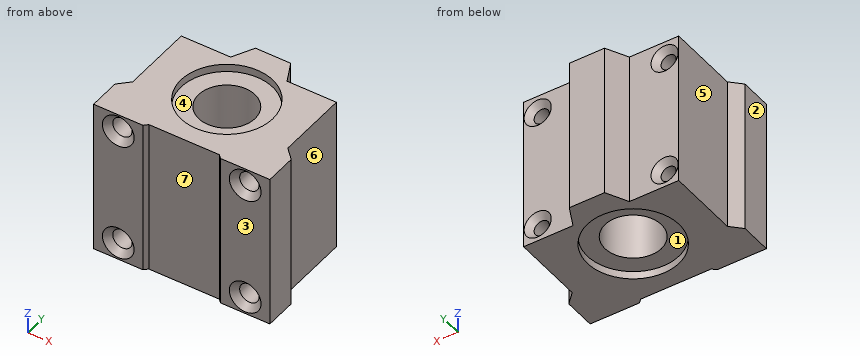
from build123d import *

# Parameters (mm, degrees)
ESBO_O1_R                                            = 8
EXTRUS_O1_DEPTH                                      = 44
ESBO_O2_R                                            = 13
EXTRUS_O2_DEPTH                                      = 2.2
ESBO_O3_R                                            = 13
EXTRUS_O3_DEPTH                                      = 2.2
ESBO_O4_R                                            = 2.15
EXTRUS_O4_DEPTH                                      = 33.5
ESCAREADO_PARA_PARAFUSO_DE_M_QUINA_COM_C_D           = 5.5
ESCAREADO_PARA_PARAFUSO_DE_M_QUINA_COM_C_DEPTH       = 12
ESCAREADO_PARA_PARAFUSO_DE_M_QUINA_COM_C_CSINK_D     = 9
ESCAREADO_PARA_PARAFUSO_DE_M_QUINA_COM_C_CSINK_ANGLE = 90
ESCAREADO_PARA_PARAFUSO_DE_M_QUINA_COM_C_TIP         = 1.652366702
CHANFRO1_SIZE                                        = 1.7


with BuildPart() as part:
    # Esboço1 → Extrusão1 (new body)
    with BuildSketch(Plane.XY):
        Polygon((-22, 13.5), (-22, -7), (-25, -10), (-25, -19), (-11, -19), (-10, -18), (10, -18), (11, -19), (25, -19), (25, -10), (22, -7), (22, 13.5), (8, 13.5), (5, 19.5), (-5, 19.5), (-8, 13.5), align=None)
        Circle(ESBO_O1_R, mode=Mode.SUBTRACT)
    extrude(amount=EXTRUS_O1_DEPTH)

    # Esboço2 → Extrusão2 (cut)
    with BuildSketch(Plane.XY.offset(44)):
        Circle(ESBO_O2_R)
    extrude(amount=-EXTRUS_O2_DEPTH, mode=Mode.SUBTRACT)

    # Esboço3 → Extrusão3 (cut)
    with BuildSketch(Plane(origin=(0, 0, 0), x_dir=(-1, 0, 0), z_dir=(0, 0, -1))):
        Circle(ESBO_O3_R)
    extrude(amount=-EXTRUS_O3_DEPTH, mode=Mode.SUBTRACT)

    # Esboço4 → Extrusão4 (cut, through all)
    with BuildSketch(Plane(origin=(0, 13.5, 0), x_dir=(1, 0, 0), z_dir=(0, 1, 0))):
        with Locations((18, -5)):
            Circle(ESBO_O4_R)
        with Locations((18, -39)):
            Circle(ESBO_O4_R)
        with Locations((-18, -5)):
            Circle(ESBO_O4_R)
        with Locations((-18, -39)):
            Circle(ESBO_O4_R)
    extrude(amount=-EXTRUS_O4_DEPTH, mode=Mode.SUBTRACT)

    # Escareado para parafuso de máquina com cabeça chata de M52
    with Locations(Plane(origin=(-18, -19, 39), x_dir=(-1, 0, 0), z_dir=(0, -1, 0))):
        with Locations((0, 0), (0, 34), (-36, 34), (-36, 0)):
            CounterSinkHole(ESCAREADO_PARA_PARAFUSO_DE_M_QUINA_COM_C_D / 2, ESCAREADO_PARA_PARAFUSO_DE_M_QUINA_COM_C_CSINK_D / 2, depth=ESCAREADO_PARA_PARAFUSO_DE_M_QUINA_COM_C_DEPTH, counter_sink_angle=ESCAREADO_PARA_PARAFUSO_DE_M_QUINA_COM_C_CSINK_ANGLE)
            with Locations((0, 0, -(ESCAREADO_PARA_PARAFUSO_DE_M_QUINA_COM_C_DEPTH + ESCAREADO_PARA_PARAFUSO_DE_M_QUINA_COM_C_TIP / 2))):  # 118° drill point
                Cone(0, ESCAREADO_PARA_PARAFUSO_DE_M_QUINA_COM_C_D / 2, ESCAREADO_PARA_PARAFUSO_DE_M_QUINA_COM_C_TIP, mode=Mode.SUBTRACT)

    # Chanfro1
    chanfro1_edges = [part.edges().sort_by_distance(p)[0] for p in [
        (15.85, 13.5, 5),
        (15.85, 13.5, 39),
        (-20.15, 13.5, 5),
        (-20.15, 13.5, 39),
    ]]
    chamfer(chanfro1_edges, length=CHANFRO1_SIZE)


solid = part.part
Part model, mm, in its own coordinate system. Face numbers are marked on the shaded views. A direction names the side the tool comes from. Round coordinates to 2 decimals unless told otherwise and drop trailing zeros. Write each loop counter-clockwise with the first axis right and the second up, starting at its lowest first coordinate (ties: lowest second). Pieces come first, ordered by that corner, then holes. Notation, with made-up numbers: M -3.75,-33 L 47.25,-33 A11 cw 47.25,-25 Z; hole C -23.75,49.5 d5. An arc over 180 degrees is marked long. Return JSON: item names as keys, results as strings. Group by question number.
(1) Saw through at C-C on z = 31. Write the cut outline in (x, y), then the cut area to 3 significant figures.
(2) Drill centre lines: probe 1 along Z at (x, y) = (18, 3); probe 2 along X at (y, z) = (-11, 39); probe 3 along X at (y, z) = (6, 5). Where is each one in solid material? Low to high.
(3) Pin check, flat tips, straight feed: pin 1 Ø1 at (x, z) = (17.5, 24.5) entering from +Y; pin 2 Ø8 at (x, y) = (18, 3.5) entering from -Z; pin 3 Ø1 at (x, y) = (11.5, -1) entering from -Z; pin 4 Ø5 at (x, z) = (-18, 39) entering from -Y. Stop position of each tip, or through.
(4) Two-plate mould, pull along Y, no slides. Class the marked faces 1, 2, 3 and 4: +Y half, -Y half, draft (parallel to the pull), parting line (faces both ways), or undercut.
(5) Saw through at A-A on y = 0. Write the cut outline in (x, z), then the cut area to 3 significant figures.
(6) Saw through at D-D on x = 0. Write the cut outline in (y, z), then the cut area to 3 significant figures.
(7) Saw through at B-B on x = 18. Write the cut outline in (y, z).
(8) Which spindle directions (+Z, -Z, +X, -X, +Y, -Y) get a long thin tool onto all of the face, cutting with end or side? Do the marked faces 5, 6 and 7. Say none if no direction does.
Returned:
{
 "1": {"outline": "M -25,-19 L -11,-19 L -10,-18 L 10,-18 L 11,-19 L 25,-19 L 25,-10 L 22,-7 L 22,13.5 L 8,13.5 L 5,19.5 L -5,19.5 L -8,13.5 L -22,13.5 L -22,-7 L -25,-10 Z; hole C 0,0 d16", "area": "1,350 mm²"},
 "2": {"probe 1": "0 to 2.85, 7.15 to 36.85, 41.15 to 44", "probe 2": "-25 to -20.75, -15.25 to 15.25, 20.75 to 25", "probe 3": "-22 to -20.15, -15.85 to -5.29, 5.29 to 15.85, 20.15 to 22"},
 "3": {"pin 1": "y = 13.5", "pin 2": "z = 0", "pin 3": "z = 2.2", "pin 4": "y = -6.85"},
 "4": {"face 1": "undercut", "face 2": "draft", "face 3": "-Y half", "face 4": "undercut"},
 "5": {"outline": "M -22,0 L -13,0 L -13,2.2 L -8,2.2 L -8,41.8 L -13,41.8 L -13,44 L -22,44 Z; M 8,2.2 L 13,2.2 L 13,0 L 22,0 L 22,44 L 13,44 L 13,41.8 L 8,41.8 Z; hole C -18,5 d4.3; hole C -18,39 d4.3; hole C 18,5 d4.3; hole C 18,39 d4.3", "area": "1,130 mm²"},
 "6": {"outline": "M -18,0 L -13,0 L -13,2.2 L -8,2.2 L -8,41.8 L -13,41.8 L -13,44 L -18,44 Z; M 8,2.2 L 13,2.2 L 13,0 L 19.5,0 L 19.5,44 L 13,44 L 13,41.8 L 8,41.8 Z", "area": "902 mm²"},
 "7": {"outline": "M -19,0 L 13.5,0 L 13.5,1.15 L 11.8,2.85 L -6.64,2.85 L -7,2.25 L -17.25,2.25 L -19,0.5 Z; M -19,9.5 L -17.25,7.75 L -7,7.75 L -6.64,7.15 L 11.8,7.15 L 13.5,8.85 L 13.5,35.15 L 11.8,36.85 L -6.64,36.85 L -7,36.25 L -17.25,36.25 L -19,34.5 Z; M -19,43.5 L -17.25,41.75 L -7,41.75 L -6.64,41.15 L 11.8,41.15 L 13.5,42.85 L 13.5,44 L -19,44 Z"},
 "8": {"face 5": "+Z, -Z, -X, +Y", "face 6": "+Z, -Z, +X, +Y", "face 7": "+Z, -Z, -Y"}
}
